Here's how the part is built. I have some questions about the finished solid (model axes, mm). A direction names the side the tool comes from. Coordinates: 2 decimals unless noted, no trailing zeros. Loops run counter-clockwise (first coordinate to the right, second up) from the corner with the lowest first, then second, coordinate; pieces in that order, holes last.
```python
from build123d import *

# Parameters (mm, degrees)
SKETCH1_W      = 3
SKETCH1_H      = 167
SKETCH2_W      = 6
SKETCH2_H      = 3
REVOLVE2_ANGLE = 3
SKETCH3_W      = 3
SKETCH3_H      = 3
REVOLVE3_ANGLE = 15


with BuildPart() as part:
    # Sketch1 → Revolve1 (revolve)
    with BuildSketch(Plane.XY, mode=Mode.PRIVATE) as revolve1_sk:
        with Locations((59.5, 83.5)):
            Rectangle(SKETCH1_W, SKETCH1_H)
    revolve(revolve1_sk.sketch.rotate(Axis((0, 0, 0), (0, 1, 0)), 90), axis=Axis((0, 0, 0), (0, 1, 0)))

    # Sketch2 → Revolve2 (revolve)
    with BuildSketch(Plane.XY):
        with Locations((-55, 165.5)):
            Rectangle(SKETCH2_W, SKETCH2_H)
        with Locations((55, 165.5)):
            Rectangle(SKETCH2_W, SKETCH2_H)
    revolve(axis=Axis((0, 0, 0), (0, 1, 0)), revolution_arc=REVOLVE2_ANGLE)

    # Sketch3 → Revolve3 (revolve)
    with BuildSketch(Plane.XY):
        with Locations((-50.5, 165.5)):
            Rectangle(SKETCH3_W, SKETCH3_H)
        with Locations((50.5, 165.5)):
            Rectangle(SKETCH3_W, SKETCH3_H)
    revolve(axis=Axis((0, 0, 0), (0, 1, 0)), revolution_arc=REVOLVE3_ANGLE)


solid = part.part
```
1. I need wall thicknesses on line 1 along X through (y, z) = (66, 0); line 2 along Z through (x, y) = (-39, 10); line 3 along X through (y, z) = (41, -49). Which ranges of each line are inside material? Lowest first, please.
2. On a 3-axis mill with a long thin cutter (end or side, diameter ignored), from which of +Z, -Z, +X, -X, +Y, -Y can I reach the whole of each face in a straight line? I mean faces 5 (the flat face through (51.55, 164, -5.33)), 6 (the flat face through (22, 0, 54)). Say none if no direction works.
3. We'd pull the mould along X, two halves only. Please class faces 1 (the flat face through (-51, 164, 5)), 2 (the flat face through (-49.4, 167, 0.3)), 3 (the cylindrical face through (59.55, 84.67, 13.22)), 4 (the cylindrical face through (51.46, 84.67, -26.76)): +X half, -X half, draft (parallel to the pull), parting line (faces both ways), or undercut.
4. I want a section at C-C (y = 80.5). Please give me the cut outline in (x, z), then the cut area to 3 significant figures.
5. I want a section at D-D (z = 8). Please give me the cut outline in (x, y).
6. For pin 1 (3 mm diameter, centred on x = 37, y = 111.5, fed in from -Z); pin 2 (4 mm diameter, centred on y = 20, z = 34.5, fed in from +X); pin 3 (5 mm diameter, centred on y = 55, z = 37, fed in from -X); pin 4 (6 mm diameter, centred on x = -40, z = 43.5, fed in from -Y), each with a flat end and sliding along its axis, tell me the tip position at first contact or that it passes through.
7. I want a section at B-B (z = 45). Please give me the cut outline in (x, y), then the cut area to 3 significant figures.
8. I want a section at A-A (x = 0). Please give me the cut outline in (y, z), then the cut area to 3 significant figures.
Response values:
1. line 1: x = -61 to -58, 58 to 61
1. line 2: z = -46.9 to -42.93, 42.93 to 46.9
1. line 3: x = -36.33 to -31.03, 31.03 to 36.33
2. face 5: -Y
2. face 6: +Z, -Z, +X, -X, -Y
3. face 1: undercut
3. face 2: draft
3. face 3: parting line
3. face 4: undercut
4. outline: circle Ø122 at (0, 0); hole circle Ø116 at (0, 0)
4. area: 1,120 mm2
5. outline: (-60.47, 0) - (-57.45, 0) - (-57.45, 167) - (-60.47, 167) - close; (-51.38, 164) - (-48.34, 164) - (-48.34, 167) - (-51.38, 167) - close; (57.45, 0) - (60.47, 0) - (60.47, 167) - (57.45, 167) - close
6. pin 1: stops at z = -49.61
6. pin 2: stops at x = 51.62
6. pin 3: stops at x = -50.31
6. pin 4: stops at y = 0
7. outline: (-41.18, 0) - (-36.59, 0) - (-36.59, 167) - (-41.18, 167) - close; (36.59, 0) - (41.18, 0) - (41.18, 167) - (36.59, 167) - close
7. area: 1,530 mm2
8. outline: (0, -61) - (167, -61) - (167, -58) - (0, -58) - close; (0, 58) - (167, 58) - (167, 61) - (0, 61) - close
8. area: 1,000 mm2
